Part print with two shaded views. Sizes in mm from the minimum x, y, z corner. A direction names the side the tool comes from. Give positions to 0.01 mm unless a question says otherwise; leave off trailing zeros. Loops run counter-clockwise (first coordinate to the right, second up) from the corner with the lowest first, then second, coordinate; pieces in that order, holes last. Notation, with made-up numbers: M 63.25,26.5 L 83.25,26.5 A13 ccw 83.25,40.5 Z; hole C 88,72 d2. An arc over 180 degrees is marked long. Answer in a Markdown table with one row per item.
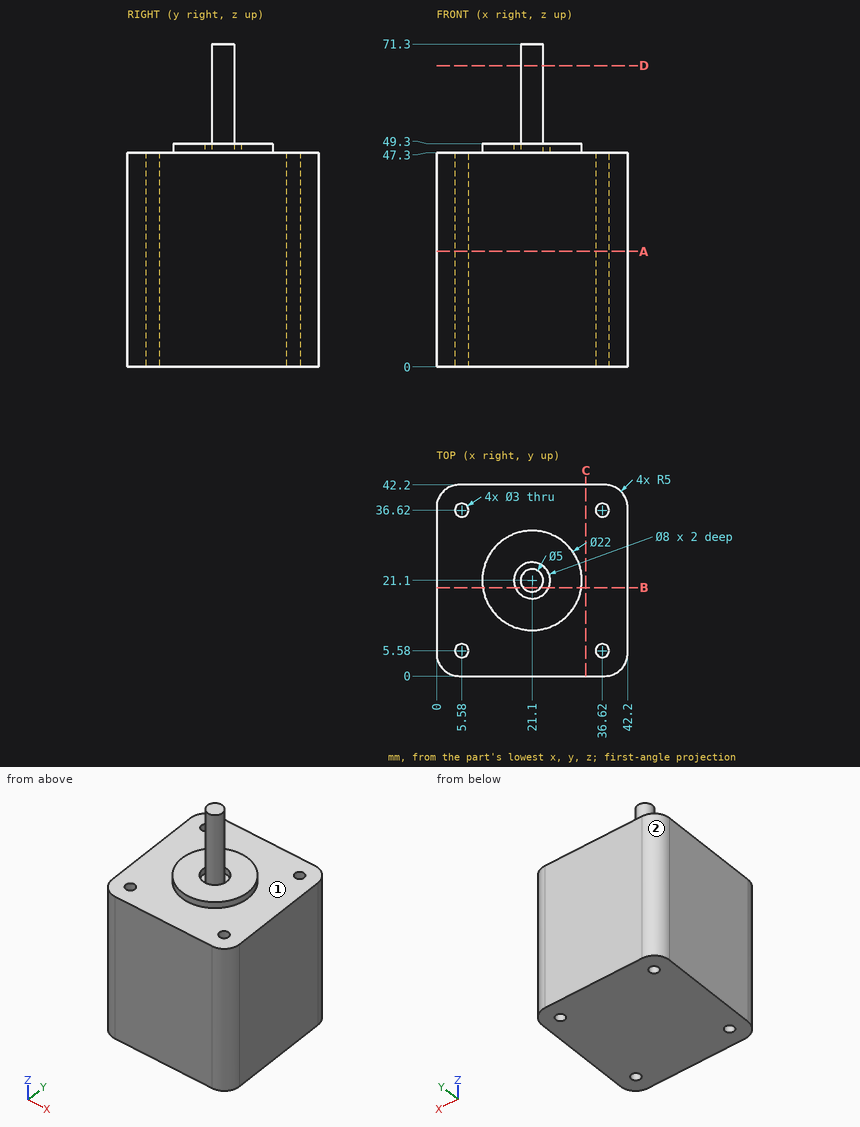
Q1. Saw through at B-B (y = 19.5). Give the cut face in (x, z).
Reported:
| item | result |
|---|---|
| outline | M 0,0 L 42.2,0 L 42.2,47.3 L 31.98,47.3 L 31.98,49.3 L 24.77,49.3 L 24.77,47.3 L 23.02,47.3 L 23.02,71.3 L 19.18,71.3 L 19.18,47.3 L 17.43,47.3 L 17.43,49.3 L 10.22,49.3 L 10.22,47.3 L 0,47.3 Z |
Q2. Drop flat-ended pins along their axis: pin 1 (5 mm diameter, centred on x = 10, y = 33.5, fed in from +Z); pin 2 (1.8 mm diameter, centred on x = 5.58, y = 5.58, fed in from -Z). Give the stop position or say it passes through.
Reported:
| item | result |
|---|---|
| pin 1 | z = 47.3 |
| pin 2 | through |
Q3. Probe probe 1 along Y at (x, z) = (5.58, 26); probe 2 along X at (y, z) = (6, 27); probe 3 along X at (y, z) = (35.5, 11.5). List the from-to ranges inside material, lowest first.
Reported:
| item | result |
|---|---|
| probe 1 | 0 to 4.08, 7.08 to 35.12, 38.12 to 42.2 |
| probe 2 | 0 to 4.14, 7.02 to 35.18, 38.06 to 42.2 |
| probe 3 | 0 to 4.58, 6.58 to 35.62, 37.62 to 42.2 |
Q4. 3-axis set-ups, long thin cutter, end or side, ignore diameter. For the marked faces 1 and 2: which of +Z, -Z, +X, -X, +Y, -Y reach the whole face in a straight line?
Reported:
| item | result |
|---|---|
| face 1 | +Z |
| face 2 | +Z, -Z, -X, +Y |
Q5. Saw through at A-A (z = 25.5). Give the cut face in (x, y).
Reported:
| item | result |
|---|---|
| outline | M 0,5 A5 ccw 5,0 L 37.2,0 A5 ccw 42.2,5 L 42.2,37.2 A5 ccw 37.2,42.2 L 5,42.2 A5 ccw 0,37.2 Z; hole C 5.58,5.58 d3; hole C 5.58,36.62 d3; hole C 36.62,5.58 d3; hole C 36.62,36.62 d3 |
Q6. Saw through at C-C (x = 33). Give the cut face in (y, z).
Reported:
| item | result |
|---|---|
| outline | M 0,0 L 42.2,0 L 42.2,47.3 L 0,47.3 Z |
Q7. Saw through at D-D (z = 66.5). Give the cut face in (x, y), and give its area (3 significant figures).
Reported:
| item | result |
|---|---|
| outline | C 21.1,21.1 d5 |
| area | 19.6 mm² |
